Input: part model. Units: mm. Frame: model coordinates. A direction names the side the tool comes from. Coordinates: 2 decimals unless noted, no trailing zeros. Write each loop counter-clockwise with the first axis right and the second up, starting at its lowest first coordinate (ties: lowest second). Pieces come first, ordered by that corner, then holes. Notation, with made-up numbers: (-38.5, 21.5) - (-9.5, 21.5) arc R12 ccw to (-9.5, 26.5) - close; hole circle Ø9 at (56, 83). An arc over 180 degrees is marked (long way). Use a Markdown table: item, result. Add a question column.
Q1. Material intervals for probe 1 along Y at (x, z) = (8, -5.5); probe 2 along Y at (x, z) = (14.5, -2.5), sorted ascending. Write a range as from..to.
Q2. Set-up query: faces 4 (the face through (4, 4, 1.8)), 5 (the face through (14.017, 13.119, 0.887)), 6 (the face through (10.398, 8.106, -5.459)). Return all of +Z, -Z, +X, -X, +Y, -Y with unobstructed straight access to the full face (end or side cutting, diameter ignored); none if empty.
Q3. Mould query, pull axis X, two halves, no side actions, for faces 1 (the face through (15, 8, -9.6)), 2 (the face through (16, 8, -5)), 3 (the face through (8, 1.2, -5)). Classes: released by +X, released by -X, zero draft, split by the parting line, or undercut.
Q4. Section query C-C (x = 11.8). Return the cut outline in (y, z).
Q5. Section query A-A (z = -7.75). Return the cut outline in (x, y).
Q6. Section query B-B (y = 8). Return the cut outline in (x, z).
Q7. Pin query (flat end, axial travel): P1, Ø3, axis at x = 8, y = 8, coming from the -Z side. Return the tip coordinate at first contact, or that it passes through.
Autodesk Inventor part; units mm, degrees
ref_plane "YZ Plane" through (0, 0, 0) normal (1, 0, 0) x (0, 1, 0)
ref_plane "XZ Plane" through (0, 0, 0) normal (0, 1, 0) x (-1, 0, 0)
ref_plane "XY Plane" through (0, 0, 0) normal (0, 0, 1) x (1, 0, 0)
sketch "Sketch1" plane through (0, 0, 0) normal (0, 0, 1) x (1, 0, 0)
  line L0 (0, 0) -> (16, 0)
  line L1 (16, 0) -> (16, 16)
  line L2 (16, 16) -> (0, 16)
  line L3 (0, 16) -> (0, 0)
  dimension "d0" = 16
  dimension "d1" = 16
extrude "Extrusion1" add sketch "Sketch1" against normal blind 9.6
sketch "Sketch2" plane through (0, 0, 0) normal (0, 0, 1) x (1, 0, 0)
  circle A0 centre (3.8, 12.2) radius 2.4
  line L0 (0, 16) -> (0, 0)
  line L1 (16, 16) -> (0, 16)
  circle A1 centre (11.8, 12.2) radius 2.4
  circle A2 centre (3.8, 4.2) radius 2.4
  circle A3 centre (11.8, 4.2) radius 2.4
  dimension "d4" = 4.8
  dimension "d5" = 3.8
  dimension "d6" = 3.8
  dimension "d7" = 4.8
  dimension "d8" = 8
  dimension "d9" = 4.8
  dimension "d10" = 4.8
  dimension "d11" = 8
extrude "Extrusion2" add sketch "Sketch2" along normal blind 1.8
sketch "Sketch3" plane through (0, 0, -9.6) normal (0, 0, -1) x (-1, 0, 0)
  line L0 (-14.8, 14.8) -> (-1.2, 14.8)
  line L1 (-1.2, 14.8) -> (-1.2, 1.2)
  line L2 (-1.2, 1.2) -> (-14.8, 1.2)
  line L3 (-14.8, 1.2) -> (-14.8, 14.8)
  line L4 (0, 16) -> (-16, 16)
  line L5 (-16, 16) -> (-16, 0)
  line L6 (-16, 0) -> (0, 0)
  line L7 (0, 16) -> (0, 0)
  circle A0 centre (-8, 8) radius 3.25
  circle A1 centre (-8, 8) radius 2.4
  dimension "d14" = 1.2
  dimension "d15" = 1.2
  dimension "d16" = 1.2
  dimension "d17" = 1.2
  dimension "d18" = 6.5
  dimension "d19" = 8
  dimension "d20" = 8
  dimension "d21" = 4.8
extrude "Extrusion3" cut sketch "Sketch3" against normal blind 8.4 contours L0 L1 L2 L3 | A1
properties part number "Yee_2x2Brick"
Values follow:
| question | item | result |
|---|---|---|
| 1 | probe 1 | 0..1.2, 4.75..5.6, 10.4..11.25, 14.8..16 |
| 1 | probe 2 | 0..1.2, 14.8..16 |
| 2 | face 4 | +Z, +X, -X, +Y, -Y |
| 2 | face 5 | +Z |
| 2 | face 6 | -Z |
| 3 | face 1 | zero draft |
| 3 | face 2 | released by +X |
| 3 | face 3 | undercut |
| 4 | outline | (0, -9.6) - (1.2, -9.6) - (1.2, -1.2) - (14.8, -1.2) - (14.8, -9.6) - (16, -9.6) - (16, 0) - (14.6, 0) - (14.6, 1.8) - (9.8, 1.8) - (9.8, 0) - (6.6, 0) - (6.6, 1.8) - (1.8, 1.8) - (1.8, 0) - (0, 0) - close |
| 5 | outline | (0, 0) - (16, 0) - (16, 16) - (0, 16) - close; circle Ø6.5 at (8, 8); hole (1.2, 1.2) - (14.8, 1.2) - (14.8, 14.8) - (1.2, 14.8) - close; hole circle Ø4.8 at (8, 8) |
| 6 | outline | (0, -9.6) - (1.2, -9.6) - (1.2, -1.2) - (4.75, -1.2) - (4.75, -9.6) - (5.6, -9.6) - (5.6, -1.2) - (10.4, -1.2) - (10.4, -9.6) - (11.25, -9.6) - (11.25, -1.2) - (14.8, -1.2) - (14.8, -9.6) - (16, -9.6) - (16, 0) - (0, 0) - close |
| 7 | P1 | z = -1.2 |
